Here's how the part is built. I have some questions about the finished solid (model axes, mm). A direction names the side the tool comes from. Give positions to 0.01 mm unless a question says otherwise; leave off trailing zeros. Order: outer loops, then holes, each group sorted by start corner. A loop starts at its lowest first (then second) coordinate and runs counter-clockwise, first axis right, second up. Notation, with made-up numbers: (39.25, 60.25) - (56.25, 60.25) arc R23 ccw to (56.25, 94.25) - close; hole circle Ø4 at (45.25, 32.5). An arc over 180 degrees is marked (long way). One line per question, with ' | ' between items.
from build123d import *

# Parameters (mm, degrees)
EXTRUDE_1_DEPTH     = 12
SKETCH_2_R          = 2.925
EXTRUDE_2_DEPTH     = 4
SKETCH_3_W          = 12.1
SKETCH_3_H          = 6.6
SKETCH_3_R          = 1.25
EXTRUDE_3_DEPTH     = 4
SKETCH_4_W          = 12.4
SKETCH_4_H          = 12
EXTRUDE_4_DEPTH     = 4
EXTRUDE_5_DEPTH     = 4
SKETCH_6_R          = 4
CUT_EXTRUDE_1_DEPTH = 4
CUT_EXTRUDE_2_DEPTH = 4
SKETCH_8_R          = 1
CUT_EXTRUDE_3_DEPTH = 1.4
CUT_EXTRUDE_4_DEPTH = 4
SKETCH_9_R          = 1.5
CUT_EXTRUDE_5_DEPTH = 5


with BuildPart() as part:
    # Sketch 1 → Extrude 1 (new body)
    with BuildSketch(Plane.XY):
        Polygon((0, 0), (25, 0), (25, 28.3), (0, 28.3), (0, 32.3), (29, 32.3), (29, -4), (0, -4), align=None)
    extrude(amount=EXTRUDE_1_DEPTH)

    # Sketch 2 → Extrude 2 (add)
    with BuildSketch(Plane.XZ.offset(4)):
        with Locations(Location((5, 6, 0), (0, 0, 90))):
            Circle(SKETCH_2_R)
    extrude(amount=EXTRUDE_2_DEPTH)

    # Sketch 3 → Extrude 3 (add)
    with BuildSketch(Plane.XY.offset(12)):
        with Locations((35.05, 29)):
            Rectangle(SKETCH_3_W, SKETCH_3_H)
        with Locations((31.6, 28.15)):
            Circle(SKETCH_3_R, mode=Mode.SUBTRACT)
        with Locations(Location((38.6, 28.15, 0), (0, 0, 180))):
            Circle(SKETCH_3_R, mode=Mode.SUBTRACT)
        with Locations((35.05, -0.7)):
            Rectangle(SKETCH_3_W, SKETCH_3_H)
        with Locations((38.6, 0.15)):
            Circle(SKETCH_3_R, mode=Mode.SUBTRACT)
        with Locations(Location((31.6, 0.15, 0), (0, 0, 180))):
            Circle(SKETCH_3_R, mode=Mode.SUBTRACT)
    extrude(amount=-EXTRUDE_3_DEPTH)

    # Sketch 4 → Extrude 4 (add)
    with BuildSketch(Plane(origin=(29, 0, 0), x_dir=(0, 0, -1), z_dir=(1, 0, 0))):
        with Locations((6.2, 19.81)):
            Rectangle(SKETCH_4_W, SKETCH_4_H)
    extrude(amount=-EXTRUDE_4_DEPTH)

    # Sketch 5 → Extrude 5 (add)
    with BuildSketch(Plane(origin=(0, 0, -12.4), x_dir=(-1, 0, 0), z_dir=(0, 0, -1))):
        with BuildLine():
            Line((-35.1, 13.81), (-25, 13.81))
            Line((-25, 13.81), (-25, 25.81))
            Line((-25, 25.81), (-35.1, 25.81))
            ThreePointArc((-35.1, 25.81), (-41.1, 19.81), (-35.1, 13.81))
        make_face()
    extrude(amount=EXTRUDE_5_DEPTH)

    # Sketch 6 → Cut-Extrude 1 (cut)
    with BuildSketch(Plane(origin=(0, 0, -16.4), x_dir=(-1, 0, 0), z_dir=(0, 0, -1))):
        with Locations((-35.1, 19.81)):
            Circle(SKETCH_6_R)
    extrude(amount=-CUT_EXTRUDE_1_DEPTH, mode=Mode.SUBTRACT)

    # Sketch 7 → Cut-Extrude 2 (cut)
    with BuildSketch(Plane(origin=(0, 32.3, 0), x_dir=(1, 0, 0), z_dir=(0, 1, 0))):
        with BuildLine():
            Line((0, -1.85), (0, -10.15))
            Line((0, -10.15), (5, -10.15))
            ThreePointArc((5, -10.15), (9.15, -6), (5, -1.85))
            Line((5, -1.85), (0, -1.85))
        make_face()
    extrude(amount=-CUT_EXTRUDE_2_DEPTH, mode=Mode.SUBTRACT)

    # Sketch 8 → Cut-Extrude 3 (cut)
    with BuildSketch(Plane(origin=(0, 32.3, 0), x_dir=(1, 0, 0), z_dir=(0, 1, 0))):
        with BuildLine():
            ThreePointArc((5.251184211, -1.857608602), (9.15, -6), (5.251184211, -10.142391398))
            Line((5.251184211, -10.142391398), (24.181578947, -8.994499806))
            ThreePointArc((24.181578947, -8.994499806), (27, -6), (24.181578947, -3.005500194))
            Line((24.181578947, -3.005500194), (5.251184211, -1.857608602))
        make_face()
        with Locations(Location((21, -6, 0), (0, 0, 270))):
            Circle(SKETCH_8_R, mode=Mode.SUBTRACT)
        with Locations(Location((18, -6, 0), (0, 0, 270))):
            Circle(SKETCH_8_R, mode=Mode.SUBTRACT)
        with Locations(Location((15, -6, 0), (0, 0, 270))):
            Circle(SKETCH_8_R, mode=Mode.SUBTRACT)
    extrude(amount=-CUT_EXTRUDE_3_DEPTH, mode=Mode.SUBTRACT)

    # Sketch 8_3 → Cut-Extrude 4 (cut)
    with BuildSketch(Plane(origin=(0, 32.3, 0), x_dir=(1, 0, 0), z_dir=(0, 1, 0))):
        with BuildLine():
            ThreePointArc((16, -6), (15, -5), (14, -6))
            Line((14, -6), (16, -6))
        make_face()
        with BuildLine():
            Line((16, -6), (14, -6))
            ThreePointArc((14, -6), (15, -7), (16, -6))
        make_face()
        with BuildLine():
            ThreePointArc((19, -6), (18, -5), (17, -6))
            Line((17, -6), (19, -6))
        make_face()
        with BuildLine():
            Line((19, -6), (17, -6))
            ThreePointArc((17, -6), (18, -7), (19, -6))
        make_face()
        with BuildLine():
            ThreePointArc((20, -6), (20.354502776, -6.763762616), (21.166666667, -6.986013297))
            ThreePointArc((21.166666667, -6.986013297), (21.041960108, -6.5), (21, -6))
            Line((21, -6), (20, -6))
        make_face()
        with BuildLine():
            ThreePointArc((21, -6), (21.041960108, -6.5), (21.166666667, -6.986013297))
            ThreePointArc((21.166666667, -6.986013297), (21.763762616, -6.645497224), (22, -6))
            Line((22, -6), (21, -6))
        make_face()
        with BuildLine():
            ThreePointArc((22, -6), (21.763762616, -5.354502776), (21.166666667, -5.013986703))
            ThreePointArc((21.166666667, -5.013986703), (21.041960108, -5.5), (21, -6))
            Line((21, -6), (22, -6))
        make_face()
        with BuildLine():
            ThreePointArc((21, -6), (21.041960108, -5.5), (21.166666667, -5.013986703))
            ThreePointArc((21.166666667, -5.013986703), (20.354502776, -5.236237384), (20, -6))
            Line((20, -6), (21, -6))
        make_face()
    extrude(amount=-CUT_EXTRUDE_4_DEPTH, mode=Mode.SUBTRACT)

    # Sketch 9 → Cut-Extrude 5 (cut)
    with BuildSketch(Plane.XZ.offset(8)):
        with Locations(Location((4.998125707, 6.006461186, 0), (0, 0, 270))):
            Circle(SKETCH_9_R)
    extrude(amount=-CUT_EXTRUDE_5_DEPTH, mode=Mode.SUBTRACT)


solid = part.part
1) I want a section at C-C (z = -3.5). List the corners of the cut face in (x, y) for me, plus the area to 3 significant figures.
Model answer:
outline: (25, 13.81) - (29, 13.81) - (29, 25.81) - (25, 25.81) - close | area: 48.0 mm2
2) Please list where these lines run through material, in increasing order: L1, parallel to Y at x = 31.6, z = 10.4; L2, parallel to Y at x = 35.1, z = -14.3; L3, parallel to Z at x = 15, y = 30.
Model answer:
L1: y = -4 to -1.1, 1.4 to 2.6, 25.7 to 26.9, 29.4 to 32.3 | L2: y = 13.81 to 15.81, 23.81 to 25.81 | L3: z = 0 to 5, 7 to 12
3) I want a section at B-B (z = -13.75). List the corners of the cut face in (x, y) for me, plus the area to 3 significant figures.
Model answer:
outline: (25, 13.81) - (35.1, 13.81) arc R6 ccw to (35.1, 25.81) - (25, 25.81) - close; hole circle Ø8 at (35.1, 19.81) | area: 127 mm2
4) I want a section at A-A (y = 19.81). List the corners of the cut face in (x, z) for me, plus the area to 3 significant figures.
Model answer:
outline: (25, -16.4) - (31.1, -16.4) - (31.1, -12.4) - (29, -12.4) - (29, 12) - (25, 12) - close; (39.1, -16.4) - (41.1, -16.4) - (41.1, -12.4) - (39.1, -12.4) - close | area: 130 mm2
5) I'm going to push flat-ended pins straight in: P1, Ø6, axis at x = 37, y = 22.5, coming from the +Z side; P2, Ø8, axis at x = 31.5, z = -6.5, coming from the -Y side; P3, Ø3, axis at x = 30.5, z = -11, coming from the +Y side; P4, Ø5, axis at x = 33.5, z = -5, coming from the -Y side. Where does each tip first touch, or does it pass through?
Model answer:
P1: stops at z = -12.4 | P2: stops at y = 13.81 | P3: stops at y = 25.81 | P4: passes through
6) I want a section at D-D (y = 4). List the corners of the cut face in (x, z) for me, plus the area to 3 significant figures.
Model answer:
outline: (25, 0) - (29, 0) - (29, 12) - (25, 12) - close | area: 48.0 mm2
7) Thinking about a two-plate mould opening in X: for faces 1 (the face through (15.5, 28.3, 4.6)), 2 (the face through (9.15, 29.88, 6.09)), 3 (the face through (3.67, -5.54, 5.31)), which applies, +X half, -X half, draft (parallel to the pull), parting line (faces both ways), or undercut?
Model answer:
face 1: draft | face 2: -X half | face 3: undercut
8) On a 3-axis mill with a long thin cutter (end or side, diameter ignored), from which of +Z, -Z, +X, -X, +Y, -Y can I reach the whole of each face in a straight line? I mean faces 4 (the face through (35, 25.7, 10)), 5 (the face through (5, -3, 6)), 6 (the face through (25, 17, 1)), 7 (the face through (27, 32, 6)). Say none if no direction works.
Model answer:
face 4: +Z, +X | face 5: -Y | face 6: +Z, -Z, -X | face 7: -X, +Y
